Study the drawing (mm; zero at the part's minimum x, y, z) and answer. Coordinates: 2 decimals unless noted, no trailing zeros. Loops run counter-clockwise (first coordinate to the right, second up) from the corner with the lowest first, then second, coordinate; pieces in that order, holes last. Notation, with made-up numbers: (-11, 19) - (-4, 19) arc R30 cw to (-4, 49) - close; hole circle Ø4 at (-0.75, -23.5). An arc over 180 degrees is marked (long way). Use one line per item in the form item = value.
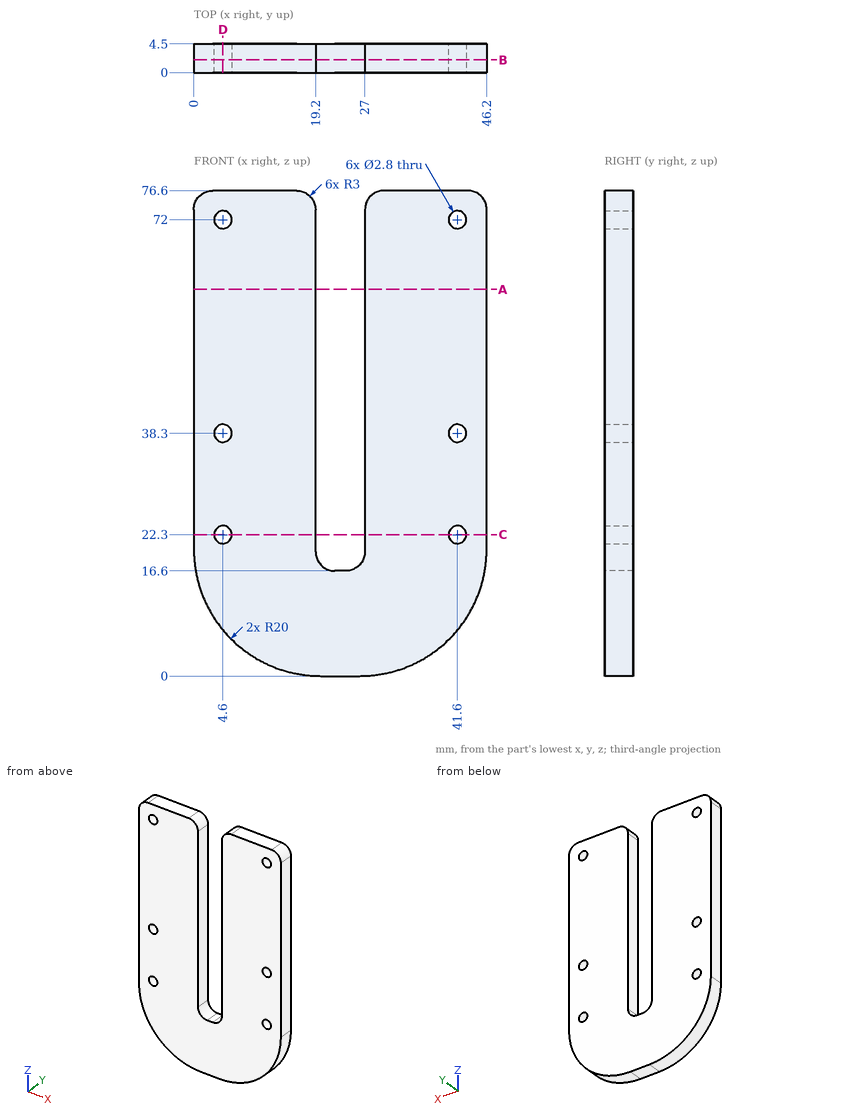
Item 1: The part is cut by section B-B on y = 2. Give the vertices of the cut face in (x, z), plus the area to 3 significant figures.
Results below:
outline = (0, 20) arc R20 ccw to (20, 0) - (26.2, 0) arc R20 ccw to (46.2, 20) - (46.2, 73.6) arc R3 ccw to (43.2, 76.6) - (30, 76.6) arc R3 ccw to (27, 73.6) - (27, 19.6) arc R3 cw to (24, 16.6) - (22.2, 16.6) arc R3 cw to (19.2, 19.6) - (19.2, 73.6) arc R3 ccw to (16.2, 76.6) - (3, 76.6) arc R3 ccw to (0, 73.6) - close; hole circle Ø2.8 at (4.6, 22.3); hole circle Ø2.8 at (4.6, 38.3); hole circle Ø2.8 at (4.6, 72); hole circle Ø2.8 at (41.6, 22.3); hole circle Ø2.8 at (41.6, 38.3); hole circle Ø2.8 at (41.6, 72)
area = 2,860 mm²
Item 2: The part is cut by section A-A on z = 61. Give the vertices of the cut face in (x, y).
Results below:
outline = (0, 0) - (19.2, 0) - (19.2, 4.5) - (0, 4.5) - close; (27, 0) - (46.2, 0) - (46.2, 4.5) - (27, 4.5) - close
Item 3: Each of these flat-tipped pins is pushed along its axis until it touches: P1, Ø0.5, axis at x = 23, y = 1.5, coming from the +Z side; P2, Ø3, axis at x = 41.6, z = 72, coming from the +Y side. Where does it stop, or does it pass through?
Results below:
P1 = 16.6
P2 = 4.5
Item 4: Find the intervals of material crossed by L1, parallel to X at y = 2.15, z = 72; L2, parallel to X at y = 4.2, z = 57.5; L3, parallel to Z at x = 4.6, y = 1.5, in increasing order.
Results below:
L1 = 0 to 3.2, 6 to 19.2, 27 to 40.2, 43 to 46.2
L2 = 0 to 19.2, 27 to 46.2
L3 = 7.24 to 20.9, 23.7 to 36.9, 39.7 to 70.6, 73.4 to 76.6
Item 5: The part is cut by section C-C on z = 22.3. Give the vertices of the cut face in (x, y).
Results below:
outline = (0, 0) - (3.2, 0) - (3.2, 4.5) - (0, 4.5) - close; (6, 0) - (19.2, 0) - (19.2, 4.5) - (6, 4.5) - close; (27, 0) - (40.2, 0) - (40.2, 4.5) - (27, 4.5) - close; (43, 0) - (46.2, 0) - (46.2, 4.5) - (43, 4.5) - close
Item 6: The part is cut by section D-D on x = 4.6. Give the vertices of the cut face in (y, z), plus the area to 3 significant figures.
Results below:
outline = (0, 7.24) - (4.5, 7.24) - (4.5, 20.9) - (0, 20.9) - close; (0, 23.7) - (4.5, 23.7) - (4.5, 36.9) - (0, 36.9) - close; (0, 39.7) - (4.5, 39.7) - (4.5, 70.6) - (0, 70.6) - close; (0, 73.4) - (4.5, 73.4) - (4.5, 76.6) - (0, 76.6) - close
area = 274 mm²
